Geometry check sheet. Reference: the model listing, model coordinates, mm. Round coordinates to 2 decimals unless told otherwise and drop trailing zeros. Order: outer loops, then holes, each group sorted by start corner. A loop starts at its lowest first (then second) coordinate and runs counter-clockwise, first axis right, second up.
```python
from build123d import *

# Parameters (mm, degrees)
F2_R = 1
F3_R = 0.3


# Not quite as in the source:
# - a feature names something its author has since deleted; it is built from what else it names


with BuildPart() as f1:
    # F0 (on Front) → F1 (revolve)
    with BuildSketch(Plane.XZ):
        Polygon((0, -70), (0, 0), (-1.4, 0), (-1.4, -1.6894261353), (-1.4, -65), align=None)
        Polygon((-1.4, -1.6894261353), (-1.4, 0), (-4, 0), (-4, -1.5247049741), align=None)
    revolve(axis=Axis((0, 0, -35), (0, 0, -1)))

    # F2
    f2_edges = [f1.edges().sort_by_distance(p)[0] for p in [
        (1.4, 0, -1.689426),
    ]]
    fillet(f2_edges, radius=F2_R)

    # F3
    f3_edges = [f1.edges().sort_by_distance(p)[0] for p in [
        (4, 0, 0),
        (4, 0, -1.524705),
    ]]
    fillet(f3_edges, radius=F3_R)


solid = f1.part
```
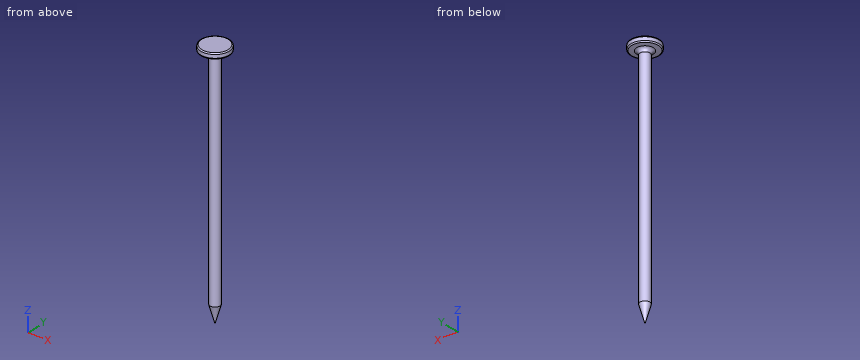
(1) Sectioned sample at A-A, the plane z = -52. Record the cut outline in (x, y), and give its area (3 significant figures).
Returned:
outline: circle Ø2.8 at (0, 0)
area: 6.16 mm2
(2) Material ranges on line 1 (Z direction, x = 2.25, y = 1); line 2 (Z direction, x = 2, y = -3); line 3 (X direction, y = -1.25, z = -36), recorded low to high.
Returned:
line 1: z = -1.62 to 0
line 2: z = -1.55 to 0
line 3: x = -0.63 to 0.63
(3) Depth check by flat-ended pin: P1, Ø1, axis at x = 1, z = -59, coming from the +Y side; P2, Ø3, axis at y = 0, z = -29, coming from the +X side. Enter the tip coordinate at first touch or a pass-through.
Returned:
P1: stops at y = 1.31
P2: stops at x = 1.4
